Autodesk Inventor part; units mm, degrees
ref_plane "YZ Plane" through (0, 0, 0) normal (1, 0, 0) x (0, 1, 0)
ref_plane "XZ Plane" through (0, 0, 0) normal (0, 1, 0) x (-1, 0, 0)
ref_plane "XY Plane" through (0, 0, 0) normal (0, 0, 1) x (1, 0, 0)
sketch "Block1" plane through (0, 0, 0) normal (0, 0, 1) x (1, 0, 0)
  line L0 (22.5674, 54.9733) -> (22.5674, 26.9733) construction
  line L1 (62.5674, 54.9733) -> (62.5674, 26.9733) construction
  line L2 (42.5674, 54.9733) -> (42.5674, 26.9733) construction
  arc A0 (22.5674, 54.9733) -> (16.0189, 31.9733) centre (39.6923, 37.6653) ccw
  arc A1 (69.116, 31.9733) -> (62.5674, 54.9733) centre (45.4425, 37.6653) ccw
  line L3 (67.5674, 31.9733) -> (69.116, 31.9733)
  line L4 (22.5674, 54.9733) -> (62.5674, 54.9733)
  arc A2 (3.175, 28.049) -> (16.0189, 31.9733) centre (7.7246, 36.1392) ccw
  arc A3 (15.3685, 38.7512) -> (3.175, 28.049) centre (13.5542, 28.5209) ccw
  arc A4 (69.116, 31.9733) -> (81.9598, 28.049) centre (77.4102, 36.1392) ccw
  arc A5 (81.9598, 28.049) -> (69.7664, 38.7512) centre (71.5807, 28.5209) ccw
  line L5 (17.5674, 54.9733) -> (67.5674, 54.9733) construction
  line L6 (67.5674, 54.9733) -> (67.5674, 31.9733) construction
  line L7 (67.5674, 31.9733) -> (16.0189, 31.9733)
  line L8 (17.5674, 31.9733) -> (17.5674, 54.9733) construction
  line L9 (22.5674, 31.9733) -> (62.5674, 31.9733)
  line L10 (62.5674, 31.9733) -> (62.5674, 26.9733)
  line L11 (62.5674, 26.9733) -> (22.5674, 26.9733)
  line L12 (22.5674, 26.9733) -> (22.5674, 31.9733)
  circle A6 centre (35.5674, 51.6287) radius 1
  circle A7 centre (49.5674, 51.6287) radius 1
  line L13 (22.5674, 29.4733) -> (62.5674, 29.4733) construction
  circle A8 centre (35.5674, 29.4733) radius 1
  circle A9 centre (49.5674, 29.4733) radius 1
  point P0 (42.5377, 37.3132)
  point P1 (42.5674, 31.9733)
  point P2 (42.5674, 31.9733)
  point P3 (17.5674, 26.9733)
  point P4 (67.5674, 26.9733)
  dimension "d0" = 23
  dimension "d1" = 5
  dimension "d2" = 40
  dimension "d3" = 2
  dimension "d4" = 2
  dimension "d5" = 7
  dimension "d6" = 7
  dimension "d7" = 2
  dimension "d8" = 2
  dimension "d9" = 7
  dimension "d10" = 7
sketch "Sketch1" plane through (0, 0, 0) normal (0, 0, 1) x (1, 0, 0)
  line L0 (-20, 11.5) -> (-20, -16.5) construction
  line L1 (20, 11.5) -> (20, -16.5) construction
  line L2 (0, 11.5) -> (0, -16.5) construction
  arc A0 (-20, 11.5) -> (-26.5485, -11.5) centre (-2.8751, -5.808) ccw
  arc A1 (26.5485, -11.5) -> (20, 11.5) centre (2.8751, -5.808) ccw
  line L3 (25, -11.5) -> (26.5485, -11.5)
  line L4 (-20, 11.5) -> (20, 11.5)
  arc A2 (-39.3924, -15.4242) -> (-26.5485, -11.5) centre (-34.8428, -7.334) ccw
  arc A3 (-27.199, -4.7221) -> (-39.3924, -15.4242) centre (-29.0132, -14.9523) ccw
  arc A4 (26.5485, -11.5) -> (39.3924, -15.4242) centre (34.8428, -7.334) ccw
  arc A5 (39.3924, -15.4242) -> (27.199, -4.7221) centre (29.0132, -14.9523) ccw
  line L5 (-25, 11.5) -> (25, 11.5) construction
  line L6 (25, 11.5) -> (25, -11.5) construction
  line L7 (25, -11.5) -> (-26.5485, -11.5)
  line L8 (-25, -11.5) -> (-25, 11.5) construction
  line L9 (-20, -11.5) -> (20, -11.5)
  line L10 (20, -11.5) -> (20, -16.5)
  line L11 (20, -16.5) -> (-20, -16.5)
  line L12 (-20, -16.5) -> (-20, -11.5)
  circle A6 centre (-7, 8.1554) radius 1
  circle A7 centre (7, 8.1554) radius 1
  line L13 (-20, -14) -> (20, -14) construction
  circle A8 centre (-7, -14) radius 1
  circle A9 centre (7, -14) radius 1
  circle A10 centre (-17, -8.5) radius 2.25
  circle A11 centre (17, -8.5) radius 2.25
  circle A12 centre (0, -8.5) radius 2.25
  line L14 (-25, 0) -> (25, 0) construction
  circle A13 centre (-7, 0) radius 1
  circle A14 centre (7, 0) radius 1
  circle A15 centre (-7, -8.1554) radius 1
  circle A16 centre (7, -8.1554) radius 1
  point P0 (0, 0)
  point P1 (0, -11.5)
  point P2 (0, -11.5)
  point P3 (-27.9814, 24.963)
  point P4 (27.9814, 24.963)
  point P5 (0, -2.5)
  point P6 (0, 0)
  dimension "d12" = 23
  dimension "d13" = 5
  dimension "d14" = 40
  dimension "d15" = 2
  dimension "d16" = 2
  dimension "d17" = 7
  dimension "d18" = 7
  dimension "d19" = 2
  dimension "d20" = 2
  dimension "d21" = 7
  dimension "d22" = 7
  dimension "d24" = 4.5
  dimension "d25" = 4.5
  dimension "d26" = 3
  dimension "d27" = 3
  dimension "d28" = 3
  dimension "d29" = 3
  dimension "d34" = 4.5
  dimension "d35" = 3
  dimension "d38" = 3.3446
  dimension "d39" = 3.3446
  dimension "d40" = 2
  dimension "d41" = 2
  dimension "d42" = 7
  dimension "d43" = 7
extrude "Extrusion1" add sketch "Sketch1" along normal blind 2 contours L4 A1 L3 L7 A0 | A10 | A11 | A12
extrude "Extrusion2" add sketch "Sketch1" along normal blind 0.6 contours A0 A2 A3
mirror "Mirror1" about plane through (0, 0, 0) normal (1, 0, 0) of "Extrusion2"
extrude "Extrusion3" cut sketch "Sketch1" along normal blind 5 contours A10 | A11 | A12
mirror "Mirror2" about plane through (0, 0, 0) normal (0, 1, 0) of "Extrusion3"
equation "\"d3\" = d11"
equation "\"d4\" = d11"
equation "\"d7\" = d11"
equation "\"d8\" = d11"
equation "\"d15\" = fishing"
equation "\"d16\" = fishing"
equation "\"d19\" = fishing"
equation "\"d20\" = fishing"
equation "\"d40\" = fishing"
equation "\"d41\" = fishing"
equation "\"d11\" = 2"
equation "\"d23\" = 2"
properties part number "Piece"
Read the model definition and answer for the solid it produces. Units are mm, in the model's axes. A direction names the side the tool comes from. Coordinates: 2 decimals unless noted, no trailing zeros. Write each loop counter-clockwise with the first axis right and the second up, starting at its lowest first coordinate (ties: lowest second). Pieces come first, ordered by that corner, then holes. Notation, with made-up numbers: (64, 39.25) -> (116, 39.25) arc R19 cw to (116, 65.25) -> close; hole circle Ø1 at (34, 4.25). An arc over 180 degrees is marked (long way). Answer as a JSON object with one key per item and string values.
Q1. The part is cut by section B-B on y = 0. Give the vertices of the cut face in (x, z), then the cut area to 3 significant figures.
The answers:
{"outline": "(-26.52, 0) -> (-8, 0) -> (-8, 2) -> (-26.52, 2) -> close; (-6, 0) -> (6, 0) -> (6, 2) -> (-6, 2) -> close; (8, 0) -> (26.52, 0) -> (26.52, 2) -> (8, 2) -> close", "area": "98.1 mm2"}
Q2. Determine the mould class of faces 3 (the flat face through (0, 11.5, 1)), 4 (the cylindrical face through (-14.854, 7.824, 0.986)) for opening direction X: pulls with the +X half, pulls with the -X half, needs draft (parallel to the pull), parting line crosses it, or undercut.
The answers:
{"face 3": "needs draft", "face 4": "undercut"}
Q3. The part is cut by section D-D on z = 1.6. Give the number of separate pieces and of enclosed holes in the cut face, then the cut area to 3 significant figures.
The answers:
{"separate pieces": "1", "enclosed holes": "12", "area": "1,060 mm2"}
Q4. Consider line 1 (Y direction, x = 7, z = 0.85); line 2 (X direction, y = -7.75, z = 0.25); line 3 (X direction, y = 0.5, z = 0.25). Determine where each line is inside the solid, lowest interval first. Write a range as [from, to].
The answers:
{"line 1": "y = [-11.5, -9.16], [-7.16, -1], [1, 7.16], [9.16, 11.5]", "line 2": "x = [-36.5, -19.12], [-14.88, -7.91], [-6.09, -2.12], [2.12, 6.09], [7.91, 14.88], [19.12, 36.5]", "line 3": "x = [-26.39, -7.87], [-6.13, 6.13], [7.87, 26.39]"}
Q5. A tool of negligible diameter and unlimited length cuts with its end or side. For faces 1 (the flat face through (0, -11.5, 1)), 2 (the flat face through (-1, -2, 0)), from which of +Z, -Z, +X, -X, +Y, -Y can it reach the whole face along a straight path? Write none if from no direction.
The answers:
{"face 1": "+Z, -Z, -Y", "face 2": "-Z, +X, -X, +Y, -Y"}
Q6. The part is cut by section A-A on x = 17. Give the vertices of the cut face in (y, z).
The answers:
{"outline": "(-11.5, 0) -> (-10.75, 0) -> (-10.75, 2) -> (-11.5, 2) -> close; (-6.25, 0) -> (6.25, 0) -> (6.25, 2) -> (-6.25, 2) -> close; (10.75, 0) -> (11.5, 0) -> (11.5, 2) -> (10.75, 2) -> close"}
Q7. Flat-ended cylindrical pins translate along their axes: pin 1 Ø1 at (y, z) = (-12, 0.5) entering from +X; pin 2 Ø2.5 at (x, y) = (-7, 0) entering from -Z; pin 3 Ø0.6 at (x, z) = (11, 1) entering from -Y; pin 4 Ø6 at (x, y) = (-30, -11.5) entering from +Z. Find the tip coordinate at first contact, or state that the pin passes through.
The answers:
{"pin 1": "stops at x = 39.11", "pin 2": "stops at z = 0", "pin 3": "stops at y = -11.5", "pin 4": "stops at z = 0.6"}
Q8. The part is cut by section C-C on y = -13. Give the vertices of the cut face in (x, z).
The answers:
{"outline": "(-39.22, 0) -> (-27.49, 0) -> (-27.49, 0.6) -> (-39.22, 0.6) -> close; (27.49, 0) -> (39.22, 0) -> (39.22, 0.6) -> (27.49, 0.6) -> close"}
